from build123d import *

# Parameters (mm, degrees)
F0_W     = 8.2
F0_H     = 10.1501198854
F3_DEPTH = 40.001


with BuildPart() as f1:
    # F0 (on Front) → F1 (revolve)
    with BuildSketch(Plane.XZ):
        with BuildLine():
            Line((0, 20.7812930996), (0, 19.9062930996))
            Line((0, 19.9062930996), (8.2, 19.9062930996))
            Line((8.2, 19.9062930996), (8.2, 9.7561732142))
            ThreePointArc((8.2, 9.7561732142), (7.5521513161, 9.157637487), (8.0976322153, 8.4645260079))
            ThreePointArc((8.0976322153, 8.4645260079), (8.1486556126, 8.4584444157), (8.2, 8.456412985))
            Line((8.2, 8.456412985), (8.2, 8.4481973997))
            Line((8.2, 8.4481973997), (8.2, -17.5937069004))
            Line((8.2, -17.5937069004), (9.9, -17.5937069004))
            Line((9.9, -17.5937069004), (9.9, -3.4926675876))
            Line((9.9, -3.4926675876), (11.4, -3.4926675876))
            Line((11.4, -3.4926675876), (11.4, 0.5073324124))
            Line((11.4, 0.5073324124), (9.9, 0.5073324124))
            Line((9.9, 0.5073324124), (9.9, 14.8537900239))
            Line((9.9, 14.8537900239), (11.4, 14.8537900239))
            Line((11.4, 14.8537900239), (11.4, 18.8537900239))
            Line((11.4, 18.8537900239), (9.9, 18.8537900239))
            Line((9.9, 18.8537900239), (9.9, 20.9062930996))
            ThreePointArc((9.9, 20.9062930996), (9.4606601718, 21.9669532714), (8.4, 22.4062930996))
            Line((8.4, 22.4062930996), (1.625, 22.4062930996))
            ThreePointArc((1.625, 22.4062930996), (1.1490485194, 21.2572445802), (0, 20.7812930996))
        make_face()
        with Locations((4.1, 14.8312331569)):
            Rectangle(F0_W, F0_H)
    revolve(axis=Axis((0, 0, 1.5937930996), (0, 0, -1)))

    # F2 (on face) → F3 (cut, through all)
    with BuildSketch(Plane.XY.offset(22.4062930996)):
        with BuildLine():
            Line((-0.7288242211, 1.4523912196), (-0.7288242211, 8.368322129))
            ThreePointArc((-0.7288242211, 8.368322129), (-5.9321762632, 5.9472081503), (-8.3664508604, 0.75))
            Line((-8.3664508604, 0.75), (-1.4415703243, 0.75))
            ThreePointArc((-1.4415703243, 0.75), (-1.1406101337, 1.1574253855), (-0.7288242211, 1.4523912196))
        make_face()
        with BuildLine():
            Line((-1.4415703243, -0.75), (-8.3664508604, -0.75))
            ThreePointArc((-8.3664508604, -0.75), (-5.9321762632, -5.9472081503), (-0.7288242211, -8.368322129))
            Line((-0.7288242211, -8.368322129), (-0.7288242211, -1.4523912196))
            ThreePointArc((-0.7288242211, -1.4523912196), (-1.1406101337, -1.1574253855), (-1.4415703243, -0.75))
        make_face()
        with BuildLine():
            ThreePointArc((0.7711757789, -8.3645255644), (5.9472098536, -5.9321745555), (8.3664508604, -0.75))
            Line((8.3664508604, -0.75), (1.4415703243, -0.75))
            ThreePointArc((1.4415703243, -0.75), (1.1574894223, -1.1405451492), (0.7711757789, -1.4303541233))
            Line((0.7711757789, -1.4303541233), (0.7711757789, -8.3645255644))
        make_face()
        with BuildLine():
            ThreePointArc((8.3664508604, 0.75), (5.9472098536, 5.9321745555), (0.7711757789, 8.3645255644))
            Line((0.7711757789, 8.3645255644), (0.7711757789, 1.4303541233))
            ThreePointArc((0.7711757789, 1.4303541233), (1.1574894223, 1.1405451492), (1.4415703243, 0.75))
            Line((1.4415703243, 0.75), (8.3664508604, 0.75))
        make_face()
    extrude(amount=-F3_DEPTH, mode=Mode.SUBTRACT)


solid = f1.part
Source: CAD feature listing. Evaluate the final solid. Frame: model axes, mm. A direction names the side the tool comes from. Coordinates: 2 decimals unless noted, no trailing zeros. Order: outer loops, then holes, each group sorted by start corner. A loop starts at its lowest first (then second) coordinate and runs counter-clockwise, first axis right, second up.
Item 1: Material intervals for line 1 (Y direction, x = 2.5, z = 20); line 2 (Y direction, x = -3.25, z = 6.5); line 3 (Z direction, x = -3.75, y = 9.25), sorted ascending.
Output values:
line 1: y = -9.58 to -8.02, -0.75 to 0.75, 8.02 to 9.58
line 2: y = -9.35 to -7.75, 7.75 to 9.35
line 3: z = -3.49 to 0.51, 14.85 to 18.85
Item 2: Cut plane A-A (z = -8.5). Return loops of the section in (x, y), plus the area to 3 significant figures.
Output values:
outline: circle Ø19.8 at (0, 0); hole (-8.37, -0.75) arc R8.4 ccw to (-0.73, -8.37) - (-0.73, -8.17) arc R8.2 ccw to (0.77, -8.16) - (0.77, -8.36) arc R8.4 ccw to (8.37, -0.75) - (8.17, -0.75) arc R8.2 ccw to (8.17, 0.75) - (8.37, 0.75) arc R8.4 ccw to (0.77, 8.36) - (0.77, 8.16) arc R8.2 ccw to (-0.73, 8.17) - (-0.73, 8.37) arc R8.4 ccw to (-8.37, 0.75) - (-8.17, 0.75) arc R8.2 ccw to (-8.17, -0.75) - close
area: 87.4 mm2
Item 3: Pull-direction query (X, two-part tool) for faces 1 (the face through (6.005, 5.874, 2.686)), 2 (the face through (0, 5, 22.406)), 3 (the face through (9.443, -2.974, 7.781)); classes: pulls with the +X half, pulls with the -X half, needs draft (parallel to the pull), parting line crosses it, or undercut.
Output values:
face 1: undercut
face 2: needs draft
face 3: parting line crosses it
Item 4: Cut plane D-D (z = -1.5). Return loops of the section in (x, y), plus the area to 3 significant figures.
Output values:
outline: circle Ø22.8 at (0, 0); hole (-8.37, -0.75) arc R8.4 ccw to (-0.73, -8.37) - (-0.73, -8.17) arc R8.2 ccw to (0.77, -8.16) - (0.77, -8.36) arc R8.4 ccw to (8.37, -0.75) - (8.17, -0.75) arc R8.2 ccw to (8.17, 0.75) - (8.37, 0.75) arc R8.4 ccw to (0.77, 8.36) - (0.77, 8.16) arc R8.2 ccw to (-0.73, 8.17) - (-0.73, 8.37) arc R8.4 ccw to (-8.37, 0.75) - (-8.17, 0.75) arc R8.2 ccw to (-8.17, -0.75) - close
area: 188 mm2
Item 5: Set-up query: faces 4 (the face through (-0.1, -10.2, 18.854)), 5 (the face through (0.1, -10.2, 14.854)), 6 (the face through (-8.2, 0, -4.8)), 7 (the face through (5.89, -5.99, 2.69)). Return all of +Z, -Z, +X, -X, +Y, -Y with unobstructed straight access to the full face (end or side cutting, diameter ignored); none if empty.
Output values:
face 4: +Z
face 5: none
face 6: -Z
face 7: +Z, -Z
Item 6: First-contact query: P1, Ø4, axis at x = 5, z = 18, coming from the +Y side; P2, Ø5, axis at x = 2.5, z = 7.5, coming from the -Y side; P3, Ø4, axis at x = 4.5, z = -4.5, coming from the -Y side. Flat tips, straight axial feed; report the tip coordinate or a pass-through.
Output values:
P1: stops at y = 11
P2: stops at y = -9.9
P3: stops at y = -11.06
Item 7: Cut plane B-B (x = 5). Count the separate pieces of the cut face and the enclosed holes in it, plus the area to 3 significant figures.
Output values:
separate pieces: 3
enclosed holes: 0
area: 189 mm2
